Geometry check sheet. Reference: the model listing, model coordinates, mm. Give positions to 0.01 mm unless a question says otherwise; leave off trailing zeros. Write each loop counter-clockwise with the first axis right and the second up, starting at its lowest first coordinate (ties: lowest second). Pieces come first, ordered by that corner, then holes.
(1) Thickness scan on line 1 along Z through (x, y) = (23.5, 52); line 2 along X through (y, z) = (23, 8.5); line 3 along X through (y, z) = (-37.5, 98.5). Record the ranges inside material, lowest first.
(2) Cross-section at C-C (z = 55). Record the boundary of the cut face in (x, y) (1 decimal), and give its area (3 significant figures).
(3) Depth check by flat-ended pin: P1, Ø7.5, axis at x = 58.08, y = 25.68, coming from the +Z side; P2, Ø2, axis at y = -9.5, z = 67.5, coming from the -X side; P3, Ø2, axis at x = -10.5, z = 82.5, coming from the -Y side; P4, Ø1.5, axis at y = -2.5, z = 84, coming from the +X side. Enter the tip coordinate at first touch or a pass-through.
(4) Cross-section at A-A (y = 0). Record the boundary of the cut face in (x, z), and give its area (3 significant figures).
(5) Cross-section at B-B (z = 10). Count the separate pieces of the cut face and the enclosed holes in it, and give its area (3 significant figures).
(6) Mould release check, pull along Z, two halves, no side actions. Record for faces 1 (the flat face through (48, -15, 16.002)), 2 (the cylindrical face through (57.62, -37.74, 101.71)), 3 (the flat face through (-1, 1, 0)), 4 (the cylindrical face through (46.94, 14.78, 54.26)): +Z half, -Z half, draft (parallel to the pull), parting line (faces both ways), or undercut.
```python
from build123d import *

# Parameters (mm, degrees)
F0_R     = 74.6125
F1_DEPTH = 16.002
F2_R     = 49.2125
F3_DEPTH = 77.597
F4_R     = 74.6125
F5_DEPTH = 16.002
F6_SIZE  = 1.27
F8_D     = 12.7
F8_DEPTH = 127


with BuildPart() as f1:
    # F0 (on Top) → F1 (new body)
    with BuildSketch(Plane.XY):
        Circle(F0_R)
    extrude(amount=F1_DEPTH)

    # F2 (on face) → F3 (join)
    with BuildSketch(Plane.XY.offset(16.002)):
        Circle(F2_R)
    extrude(amount=F3_DEPTH)

    # F4 (on face) → F5 (join)
    with BuildSketch(Plane.XY.offset(93.599)):
        Circle(F4_R)
    extrude(amount=F5_DEPTH)

    # F6
    f6_edges = [f1.edges().sort_by_distance(p)[0] for p in [
        (-74.6125, 0, 93.599),
        (-74.6125, 0, 109.601),
        (-74.6125, 0, 16.002),
        (-74.6125, 0, 0),
    ]]
    chamfer(f6_edges, length=F6_SIZE)

    # F8
    with Locations(Plane(origin=(0, 0, 0), x_dir=(1, 0, 0), z_dir=(0, 0, -1))):
        with Locations((-51.276663, -37.456026), (-58.076201, 25.67888), (-6.799538, 63.134905), (51.276663, 37.456026), (58.076201, -25.67888), (6.799538, -63.134905)):
            Hole(F8_D / 2, depth=F8_DEPTH)


solid = f1.part
```
Reply:
1. line 1: z = 0 to 16, 93.6 to 109.6
1. line 2: x = -70.98 to 52.32, 63.83 to 70.98
1. line 3: x = -64.5 to 44.93, 57.63 to 64.5
2. outline: circle Ø98.4 at (0, 0)
2. area: 7,610 mm2
3. P1: passes through
3. P2: stops at x = -48.47
3. P3: stops at y = -48.29
3. P4: stops at x = 49.18
4. outline: (-74.61, 1.27) - (-73.34, 0) - (73.34, 0) - (74.61, 1.27) - (74.61, 14.73) - (73.34, 16) - (49.21, 16) - (49.21, 93.6) - (73.34, 93.6) - (74.61, 94.87) - (74.61, 108.33) - (73.34, 109.6) - (-73.34, 109.6) - (-74.61, 108.33) - (-74.61, 94.87) - (-73.34, 93.6) - (-49.21, 93.6) - (-49.21, 16) - (-73.34, 16) - (-74.61, 14.73) - close
4. area: 12,400 mm2
5. separate pieces: 1
5. enclosed holes: 6
5. area: 16,700 mm2
6. face 1: undercut
6. face 2: draft
6. face 3: -Z half
6. face 4: undercut
